Read the model definition and answer for the solid it produces. Units are mm, in the model's axes. A direction names the side the tool comes from. Round coordinates to 2 decimals unless told otherwise and drop trailing zeros. Write each loop counter-clockwise with the first axis right and the second up, starting at its lowest first coordinate (ties: lowest second). Pieces come first, ordered by that corner, then holes. Notation, with made-up numbers: (-35, 68) - (24, 68) arc R21 cw to (24, 92) - close; hole circle Ø9 at (-26.75, 28). An arc over 180 degrees is marked (long way). One line per item, written item: value. Start each with the question number.
(1) The mould has two halves that part along X. Classify faces 3 (the face through (-21.92, -6.2, 30.99)), 4 (the face through (-29.403, -1.566, -9.269)): +X half, -X half, draft (parallel to the pull), parting line (faces both ways), or undercut.
(2) For faces 1 (the face through (-29.88, -14.96, 30.1)), 2 (the face through (-21.5, -11, -2)), determine the directions among +Z, -Z, +X, -X, +Y, -Y from which every point of the face is accessible in a straight line to the end or side of a thin tool.
(3) A cutting plane is placed at A-A, the plane z = 17.5. Determine the outline of the cut face in (x, y).
(4) A flat-ended cylindrical pin translates along its axis: pin 1 Ø2.5 at (x, z) = (-16.6, -9.9) entering from +Y. Find the tip coordinate at first contact, or state that the pin passes through.
(5) A cutting plane is placed at C-C, the plane x = -15.5. Determine the outline of the cut face in (y, z), plus the area to 3 significant figures.
(6) A cutting plane is placed at D-D, the plane z = 23. Determine the outline of the cut face in (x, y), plus the area to 3 significant figures.
(7) A cutting plane is placed at B-B, the plane x = -23.25. Determine the outline of the cut face in (y, z).
(8) Find the intervals of material crossed by L1, parallel to Z at x = -23, y = -4.1; L2, parallel to Z at x = -30.5, y = -4.1; L3, parallel to Y at x = -13.9, z = -9.9, in increasing order.
from build123d import *

# Parameters (mm, degrees)
F0_W     = 19
F0_H     = 49
F0_W_2   = 9
F0_H_2   = 21
F1_DEPTH = 21
F2_W     = 1
F2_H     = 4
F3_DEPTH = 25
F4_R     = 2.1
F5_DEPTH = 25
F6_R     = 2.1
F7_DEPTH = 25


with BuildPart() as f1:
    # F0 (on Front) → F1 (new body)
    with BuildSketch(Plane.XZ):
        with Locations((-21.999743, 10.5)):
            Rectangle(F0_W, F0_H)
        with Locations((-21.999743, 10.5)):
            Rectangle(F0_W_2, F0_H_2, mode=Mode.SUBTRACT)
    extrude(amount=F1_DEPTH)

    # F2 (on face) → F3 (cut)
    with BuildSketch(Plane.XZ.offset(21)):
        with Locations((-21.999743, 23)):
            Rectangle(F2_W, F2_H)
        with Locations((-21.999743, -2)):
            Rectangle(F2_W, F2_H)
    extrude(amount=-F3_DEPTH, mode=Mode.SUBTRACT)

    # F4 (on face) → F5 (cut)
    with BuildSketch(Plane(origin=(0, 0, 0), x_dir=(-1, 0, 0), z_dir=(0, 1, 0))):
        with Locations((16.599743, 30.9)):
            Circle(F4_R)
        with Locations((16.599743, -9.9)):
            Circle(F4_R)
        with Locations((27.399743, -9.9)):
            Circle(F4_R)
        with Locations((27.399743, 30.9)):
            Circle(F4_R)
    extrude(amount=-F5_DEPTH, mode=Mode.SUBTRACT)

    # F6 (on face) → F7 (cut)
    with BuildSketch(Plane.YZ.offset(-12.499743)):
        with Locations((-16.9, 30.9)):
            Circle(F6_R)
        with Locations((-16.9, -9.9)):
            Circle(F6_R)
        with Locations((-4.1, 30.9)):
            Circle(F6_R)
        with Locations((-4.1, -9.9)):
            Circle(F6_R)
    extrude(amount=-F7_DEPTH, mode=Mode.SUBTRACT)


solid = f1.part
Here are the results:
1. face 3: draft
1. face 4: undercut
2. face 1: +X, -X
2. face 2: +Y, -Y
3. outline: (-31.5, -21) - (-26.5, -21) - (-26.5, 0) - (-31.5, 0) - close; (-17.5, -21) - (-12.5, -21) - (-12.5, 0) - (-17.5, 0) - close
4. pin 1: through
5. outline: (-21, -14) - (0, -14) - (0, -11.69) - (-3, -11.69) arc R2.1 cw to (-5.2, -11.69) - (-15.8, -11.69) arc R2.1 cw to (-18, -11.69) - (-21, -11.69) - close; (-21, -8.11) - (-18, -8.11) arc R2.1 cw to (-15.8, -8.11) - (-5.2, -8.11) arc R2.1 cw to (-3, -8.11) - (0, -8.11) - (0, 29.11) - (-3, 29.11) arc R2.1 cw to (-5.2, 29.11) - (-15.8, 29.11) arc R2.1 cw to (-18, 29.11) - (-21, 29.11) - close; (-21, 32.69) - (-18, 32.69) arc R2.1 cw to (-15.8, 32.69) - (-5.2, 32.69) arc R2.1 cw to (-3, 32.69) - (0, 32.69) - (0, 35) - (-21, 35) - close
5. area: 875 mm²
6. outline: (-31.5, -21) - (-22.5, -21) - (-22.5, 0) - (-31.5, 0) - close; (-21.5, -21) - (-12.5, -21) - (-12.5, 0) - (-21.5, 0) - close
6. area: 378 mm²
7. outline: (-21, -14) - (0, -14) - (0, 0) - (-21, 0) - close; (-21, 21) - (0, 21) - (0, 35) - (-21, 35) - close; hole circle Ø4.2 at (-16.9, -9.9); hole circle Ø4.2 at (-16.9, 30.9); hole circle Ø4.2 at (-4.1, -9.9); hole circle Ø4.2 at (-4.1, 30.9)
8. L1: -14 to -12, -7.8 to 0, 21 to 28.8, 33 to 35
8. L2: -14 to -12, -7.8 to 28.8, 33 to 35
8. L3: -21 to -19, -14.8 to -6.2, -2 to 0
